from build123d import *

# Parameters (mm, degrees)
F1_DEPTH = 0.889
F3_DEPTH = 152.4
F5_DEPTH = 4.318


with BuildPart() as f1:
    # F0 (on Top) → F1 (new body)
    with BuildSketch(Plane.XY):
        with BuildLine():
            ThreePointArc((73.319457, 74.928008), (53.181192, 129.299909), (0, 152.4))
            ThreePointArc((0, 152.4), (-152.4, 0), (0, -152.4))
            ThreePointArc((0, -152.4), (47.743568, -42.310835), (73.319457, 74.928008))
        make_face()
    extrude(amount=F1_DEPTH)

    # F2 (on face) → F3 (join)
    with BuildSketch(Plane(origin=(0, 0, 0), x_dir=(1, 0, 0), z_dir=(0, 0, -1))):
        with BuildLine():
            Line((0.001841, 152.457275), (0, 152.4))
            ThreePointArc((0, 152.4), (0.431777, 151.620209), (0.862429, 150.839797))
            ThreePointArc((0.862429, 150.839797), (1.545113, 157.643166), (-3.264828, 152.7835))
            Line((-3.264828, 152.7835), (-1.715005, 153.532948))
            ThreePointArc((-1.715005, 153.532948), (1.011435, 155.976592), (0.001841, 152.457275))
        make_face()
        with BuildLine():
            ThreePointArc((0.862429, 150.839797), (0.431777, 151.620209), (0, 152.4))
            ThreePointArc((0, 152.4), (-141.177371, 57.399564), (-106.345401, -109.162337))
            Line((-106.345401, -109.162337), (-105.184084, -107.970258))
            ThreePointArc((-105.184084, -107.970258), (-139.635681, 56.772747), (0, 150.735756))
            ThreePointArc((0, 150.735756), (0.434341, 150.76186), (0.862429, 150.839797))
        make_face()
    extrude(amount=F3_DEPTH)

    # F4 (on Right) → F5 (cut, symmetric)
    with BuildSketch(Plane.YZ):
        Polygon((-151.658967, 0), (-150.745168, 0), (-150.745168, 1.181528), (-161.246374, 1.181528), (-161.246374, 0), (-165.631473, 0), (-165.631473, -152.882606), (-161.246374, -152.882606), (-161.246374, -126.9674), (-151.658967, -126.9674), (-151.658967, -101.560883), (-161.246374, -101.560883), (-161.246374, -76.169804), (-151.658967, -76.169804), (-151.658967, -50.782207), (-161.246374, -50.782207), (-161.246374, -25.388533), (-151.658967, -25.388533), align=None)
    extrude(amount=F5_DEPTH, both=True, mode=Mode.SUBTRACT)


solid = f1.part
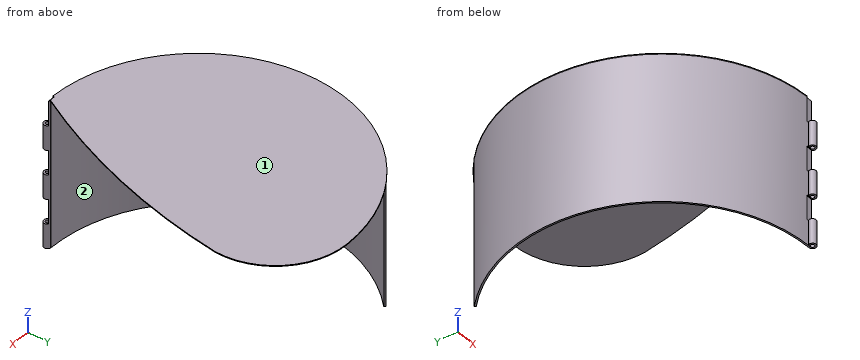
The model under review builds one solid part; all positions refer to its coordinate system, in mm. Face numbers are marked on the shaded views. Coordinates: 2 decimals unless noted, no trailing zeros. Loops run counter-clockwise (first coordinate to the right, second up) from the corner with the lowest first, then second, coordinate; pieces in that order, holes last.
(1) Insertion check: P1, Ø7, axis at x = 0, y = -154.5, coming from the +Z side; P2, Ø5, axis at x = 1.5, y = -154, coming from the -Z side; P3, Ø2, axis at x = -2, z = -108.5, coming from the -Y side; P4, Ø5, axis at x = -64, z = -55.5, coming from the -Y side. Each pin has a flat end and moves straight along its axis. Give the tip position at first contact, or say it passes through.
Determined:
P1: stops at z = 0
P2: stops at z = -152.4
P3: stops at y = -151.66
P4: stops at y = -139.44
(2) Consider section D-D, the plane x = 39. Give the boundary of the cut face in (y, z), plus the area to 3 significant figures.
Determined:
outline: (-67.54, 0) - (140.97, 0) - (140.97, 0.89) - (-67.54, 0.89) - close
area: 185 mm2
(3) Draft analysis for pull direction Y (two halves, no side actions). For the marked faces 1 and 2, state which applies: +Y half, -Y half, draft (parallel to the pull), parting line (faces both ways), or undercut.
Determined:
face 1: draft
face 2: undercut
(4) Wall thickness on L1, parallel to Z at x = 35, y = 123; L2, parallel to Y at x = -113.5, z = -94.5; L3, parallel to Y at x = -132.5, z = -49: over which ranges is each line inside the solid? List them lowest first.
Determined:
L1: z = 0 to 0.89
L2: y = -101.7 to -99.19, 99.19 to 101.7
L3: y = -75.3 to -71.87, 71.87 to 75.3
(5) Consider section B-B, the plane x = -96.5. Give the boundary of the cut face in (y, z), plus the area to 3 significant figures.
Determined:
outline: (-117.96, -152.4) - (-115.8, -152.4) - (-115.8, 0) - (117.96, 0) - (117.96, 0.89) - (-117.96, 0.89) - close
area: 539 mm2
(6) Consider section A-A, the plane z = -122.5. Give the boundary of the cut face in (x, y), plus the area to 3 significant figures.
Determined:
outline: (-106.35, 109.16) arc R152.4 ccw to (-4.32, -152.34) - (-4.32, -151.66) - (2.42, -151.66) arc R3.63 ccw to (0.86, -150.84) arc R3.63 ccw to (0, -150.74) arc R150.74 cw to (-105.18, 107.97) - close
area: 596 mm2
